Check sheet for the modelled part. Datum: model origin and axes. Units: mm. Face numbers are marked on the shaded views. A direction names the side the tool comes from. Coordinates: 2 decimals unless noted, no trailing zeros. Loops run counter-clockwise (first coordinate to the right, second up) from the corner with the lowest first, then second, coordinate; pieces in that order, holes last. Notation, with made-up numbers: (81.25, -18.75) -> (128.25, -18.75) arc R20 ccw to (128.25, -10.75) -> close; hole circle Ø1 at (40.5, -2.75). An arc over 180 degrees is marked (long way). Use one line per item in the form item = value.
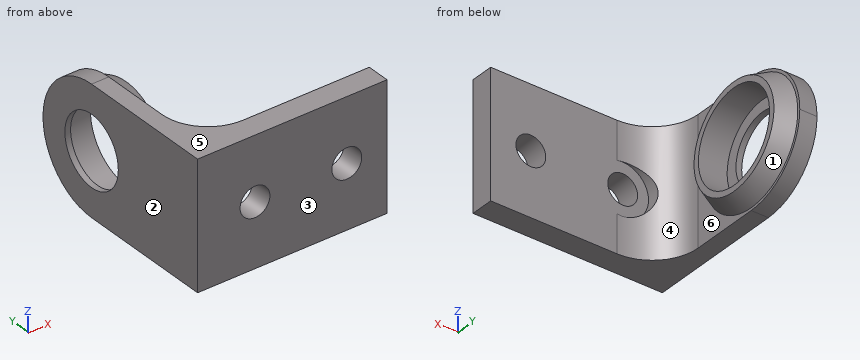
Autodesk Inventor part; units mm, degrees
ref_plane "YZ Plane" through (0, 0, 0) normal (1, 0, 0) x (0, 1, 0)
ref_plane "XZ Plane" through (0, 0, 0) normal (0, 1, 0) x (-1, 0, 0)
ref_plane "XY Plane" through (0, 0, 0) normal (0, 0, 1) x (1, 0, 0)
sketch "Sketch3" plane through (0, 0, 0) normal (0, 0, 1) x (1, 0, 0)
  line L0 (0, 0) -> (0, 35)
  line L1 (0, 35) -> (3, 35)
  line L2 (3, 35) -> (3, 4)
  line L3 (3, 4) -> (33, 4)
  line L4 (33, 4) -> (33, 0)
  line L5 (33, 0) -> (0, 0)
  line L6 (0, 25) -> (3, 25) construction
  dimension "d0" = 10
  dimension "d1" = 25
  dimension "d2" = 30
  dimension "d3" = 4
  dimension "d4" = 3
extrude "Extrusion1" add sketch "Sketch3" along normal mid plane 22
sketch "Sketch4" plane through (3, 4, -11) normal (1, 0, 0) x (0, 0, -1)
  line L0 (0, 31) -> (-22, 31) construction
  line L1 (-11, 31) -> (-11, 20) construction
  circle A0 centre (-11, 20) radius 8.05
  point P0 (-11, -4)
  dimension "d7" = 11
  dimension "d8" = 16.1
extrude "Extrusion2" cut sketch "Sketch4" against normal through all
fillet "Fillet3" radius 8 1 edges at (3, 4, 0)
sketch "Sketch5" plane through (3, 4, -11) normal (0, 1, 0) x (1, 0, 0)
  line L0 (30, 0) -> (30, -22) construction
  line L1 (30, -11) -> (0, -11) construction
  line L2 (0, 0) -> (0, -22) construction
  circle A0 centre (7, -11) radius 2.6
  circle A1 centre (23, -11) radius 2.6
  point P0 (-3, -11)
  dimension "d11" = 7
  dimension "d12" = 7
  dimension "d13" = 5.2
extrude "Extrusion3" cut sketch "Sketch5" along normal mid plane 24.75
sketch "Sketch6" plane through (0, 0, 0) normal (0, 0, 1) x (1, 0, 0)
  line L0 (3, 15.95) -> (0, 15.95) construction
  line L1 (0, 15.95) -> (0, 17.95)
  line L2 (0, 17.95) -> (1, 17.95)
  line L3 (1, 17.95) -> (1, 15.95)
  line L4 (0, 15.95) -> (0, 32.05) construction
  line L5 (1, 15.95) -> (0, 15.95)
  line L6 (3, 32.05) -> (3, 15.95) construction
  line L7 (3, 15.95) -> (6, 15.95)
  line L8 (6, 15.95) -> (6, 14.95)
  line L9 (6, 14.95) -> (3, 13.45)
  line L10 (3, 13.45) -> (3, 15.95)
  line L11 (0, 24) -> (3, 24) construction
  point P0 (0, 0)
  dimension "d16" = 1
  dimension "d17" = 2
  dimension "d18" = 5
  dimension "d19" = 2.5
  dimension "d20" = 1
revolve "Revolution1" add sketch "Sketch6" angle 360 about axis through (0, 24, 0) along (1, 0, 0)
fillet "Fillet1" radius 11 2 edges at (1.5, 35, 11) (1.5, 35, -11)
sketch "Sketch11" plane through (33, 4, 11) normal (0, 1, 0) x (1, 0, 0)
  circle A0 centre (-23, 11) radius 2.6
  circle A1 centre (-23, 11) radius 4.5
  point P0 (-33, 11)
  dimension "d42" = 9
extrude "Extrusion8" cut sketch "Sketch11" along normal blind 5 contours A0 | A1
properties part number "Winder_idler"
(1) Scan lines: line 1 along X through (y, z) = (1, 0); line 2 along Y through (x, z) = (3.8, 0); line 3 along Y through (x, z) = (4.5, -6.5). Record each from-to range of solid material in increasing order.
Established:
line_1 = 0 to 7.4, 12.6 to 23.4, 28.6 to 33
line_2 = 0 to 8.51, 13.85 to 15.95, 32.05 to 34.15
line_3 = 0 to 7.34, 16.67 to 19.25, 28.75 to 31.33
(2) Section check C-C, the plane x = 20.5. Record the boundary of the cut face in (y, z), plus the area to 3 significant figures.
Established:
outline = (0, -11) -> (4, -11) -> (4, 11) -> (0, 11) -> close
area = 88.0 mm²
(3) Go/stop test with flat-tipped pins: P1, Ø11, axis at y = 24, z = 0, coming from the -X side; P2, Ø4, axis at x = 18, z = 6, coming from the +Y side; P3, Ø13, axis at y = 24.5, z = -2, coming from the +X side. Record where each tip stops, or that it passes through.
Established:
P1 = through
P2 = 4
P3 = 6
(4) Section check A-A, the plane x = 26. Record the boundary of the cut face in (y, z).
Established:
outline = (0, -11) -> (4, -11) -> (4, -2.6) -> (0, -2.6) -> close; (0, 2.6) -> (4, 2.6) -> (4, 11) -> (0, 11) -> close
(5) Mould release check, pull along Y, two halves, no side actions. Record for the marked faces 1, 2 and 3: +Y half, -Y half, draft (parallel to the pull), parting line (faces both ways), or undercut.
Established:
face_1 = undercut
face_2 = draft
face_3 = -Y half
(6) Tool access check on the marked faces 4, 5 and 6. Record the directions out of +Z, -Z, +X, -X, +Y, -Y that give a thin tool (end or side, any length) a straight path to the whole face; none if there is none.
Established:
face_4 = +Z, -Z, +X
face_5 = +Z, +X, -X, +Y, -Y
face_6 = +X
(7) Section check B-B, the plane x = 10. Record the boundary of the cut face in (y, z).
Established:
outline = (0, -11) -> (4.06, -11) -> (4.06, -4.5) -> (4, -4.5) -> (4, -2.6) -> (0, -2.6) -> close; (0, 2.6) -> (4, 2.6) -> (4, 4.5) -> (4.06, 4.5) -> (4.06, 11) -> (0, 11) -> close
(8) Section check D-D, the plane z = 0.5. Give the number of separate pieces and of enclosed holes in the cut face, plus the area to 3 significant figures.
Established:
separate_pieces = 4
enclosed_holes = 0
area = 160 mm²
